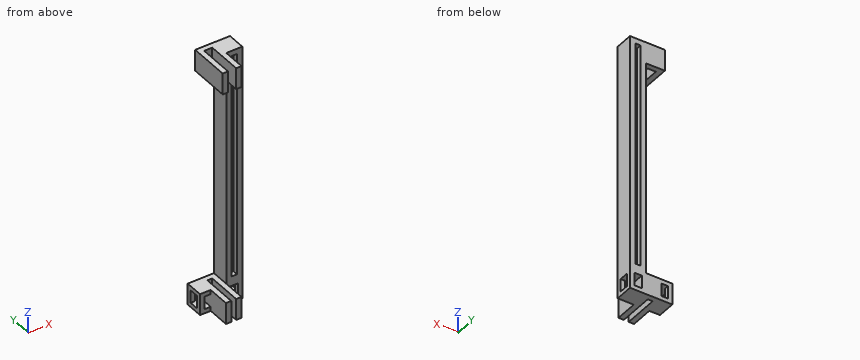
from build123d import *

# Parameters (mm, degrees)
F1_DEPTH  = 10
F2_W      = 7.5
F2_H      = 8.5
F3_DEPTH  = 110.255
F5_DEPTH  = 10
F6_W      = 4.5
F6_H      = 6
F7_DEPTH  = 5
F8_W      = 3
F8_H      = 6
F9_DEPTH  = 8.501
F10_W     = 4.5
F10_H     = 6
F11_DEPTH = 5
F12_W     = 3.5
F12_H     = 6
F13_DEPTH = 8.501
F14_W     = 2.5
F14_H     = 105.255
F15_DEPTH = 2.5
F16_W     = 2.5
F16_H     = 105.255
F17_DEPTH = 2.5


with BuildPart() as f1:
    # F0 (on Top) → F1 (new body)
    with BuildSketch(Plane.XY):
        Polygon((0, -8.5), (0, 0), (-19.8, 0), (-19.8, -8.5), (-14.8, -8.5), (-14.8, -19), (-12.3, -19), (-12.3, -2.5), (-10, -2.5), (-10, -19), (-7.5, -19), (-7.5, -8.5), align=None)
    extrude(amount=F1_DEPTH)

    # F2 (on face) → F3 (join)
    with BuildSketch(Plane.XY.offset(10)):
        with Locations((-3.75, -4.25)):
            Rectangle(F2_W, F2_H)
    extrude(amount=F3_DEPTH)

    # F4 (on face) → F5 (join)
    with BuildSketch(Plane.XY.offset(120.255)):
        Polygon((-7.5, -19), (-7.5, 0), (-16.3, 0), (-16.3, -19), (-13.8, -19), (-13.8, -2.5), (-10, -2.5), (-10, -19), align=None)
    extrude(amount=-F5_DEPTH)

    # F6 (on face) → F7 (cut, through all)
    with BuildSketch(Plane(origin=(-19.8, 0, 0), x_dir=(0, -1, 0), z_dir=(-1, 0, 0))):
        with Locations((4.25, 5)):
            Rectangle(F6_W, F6_H)
    extrude(amount=-F7_DEPTH, mode=Mode.SUBTRACT)

    # F8 (on face) → F9 (cut, through all)
    with BuildSketch(Plane.XZ.offset(8.5)):
        with Locations((-16.3, 5)):
            Rectangle(F8_W, F8_H)
    extrude(amount=-F9_DEPTH, mode=Mode.SUBTRACT)

    # F10 (on face) → F11 (cut)
    with BuildSketch(Plane.YZ):
        with Locations((-4.25, 5)):
            Rectangle(F10_W, F10_H)
    extrude(amount=-F11_DEPTH, mode=Mode.SUBTRACT)

    # F12 (on face) → F13 (cut, through all)
    with BuildSketch(Plane.XZ.offset(8.5)):
        with Locations((-3.75, 5)):
            Rectangle(F12_W, F12_H)
    extrude(amount=-F13_DEPTH, mode=Mode.SUBTRACT)

    # F14 (on face) → F15 (cut)
    with BuildSketch(Plane(origin=(0, 0, 0), x_dir=(-1, 0, 0), z_dir=(0, 1, 0))):
        with Locations((3.75, 65.1275)):
            Rectangle(F14_W, F14_H)
    extrude(amount=-F15_DEPTH, mode=Mode.SUBTRACT)

    # F16 (on face) → F17 (cut)
    with BuildSketch(Plane.XZ.offset(8.5)):
        with Locations((-3.75, 65.1275)):
            Rectangle(F16_W, F16_H)
    extrude(amount=-F17_DEPTH, mode=Mode.SUBTRACT)


solid = f1.part
Part model, mm, in its own coordinate system. Coordinates: 2 decimals unless noted, no trailing zeros. Loops run counter-clockwise (first coordinate to the right, second up) from the corner with the lowest first, then second, coordinate; pieces in that order, holes last. Notation, with made-up numbers: (87, 50) -> (99, 50) arc R27 ccw to (99, 71) -> close; hole circle Ø3 at (-16, 63.25). An arc over 180 degrees is marked (long way). Use a Markdown table: item, result. Add a question column.
Item 1: Flat gauge pins, fed straight in: P1, Ø8, axis at x = -3.5, z = 107.5, coming from the -Y side; P2, Ø9.5, axis at y = -5.5, z = 57, coming from the -X side; P3, Ø1.2, axis at x = -4, z = 67.5, coming from the +Y side. Where does each tip first touch, or does it go through?
Item 2: Band-saw the part on C-C on z = 81. Write the cut outline in (x, y).
Item 3: Band-saw the part on A-A on y = -9.5. Write the cut outline in (x, z) (3 decimals).
Item 4: Band-saw the part on B-B on x = -9. Write the cut outline in (y, z) (3 decimals).
Item 5: Probe probe 1 along Z at (x, y) = (-8.5, -18) (3 decimals); probe 2 along X at (y, z) = (-8.25, 6.5); probe 3 along X at (y, z) = (-11.75, 111). List the from-to ranges inside material, lowest first.
Geometry says:
| question | item | result |
|---|---|---|
| 1 | P1 | y = -8.5 |
| 1 | P2 | x = -7.5 |
| 1 | P3 | y = -2.5 |
| 2 | outline | (-7.5, -8.5) -> (-5, -8.5) -> (-5, -6) -> (-2.5, -6) -> (-2.5, -8.5) -> (0, -8.5) -> (0, 0) -> (-2.5, 0) -> (-2.5, -2.5) -> (-5, -2.5) -> (-5, 0) -> (-7.5, 0) -> close |
| 3 | outline | (-16.3, 110.255) -> (-13.8, 110.255) -> (-13.8, 120.255) -> (-16.3, 120.255) -> close; (-14.8, 0) -> (-12.3, 0) -> (-12.3, 10) -> (-14.8, 10) -> close; (-10, 0) -> (-7.5, 0) -> (-7.5, 10) -> (-10, 10) -> close; (-10, 110.255) -> (-7.5, 110.255) -> (-7.5, 120.255) -> (-10, 120.255) -> close |
| 4 | outline | (-19, 0) -> (0, 0) -> (0, 10) -> (-19, 10) -> close; (-19, 110.255) -> (0, 110.255) -> (0, 120.255) -> (-19, 120.255) -> close |
| 5 | probe 1 | 0 to 10, 110.255 to 120.255 |
| 5 | probe 2 | -19.8 to -17.8, -14.8 to -12.3, -10 to -5.5, -2 to 0 |
| 5 | probe 3 | -16.3 to -13.8, -10 to -7.5 |
